Here's the drawing with two shaded views (mm, measured from the low corner). I have some questions. Coordinates: 2 decimals unless noted, no trailing zeros. Loops run counter-clockwise (first coordinate to the right, second up) from the corner with the lowest first, then second, coordinate; pieces in that order, holes last. Notation, with made-up numbers: M 70.25,7.25 L 80.25,7.25 A13 ccw 80.25,21.25 Z; hole C 38,5 d4. An arc over 180 degrees is marked long. Return JSON: item names as keys, results as strings. Group by question number.
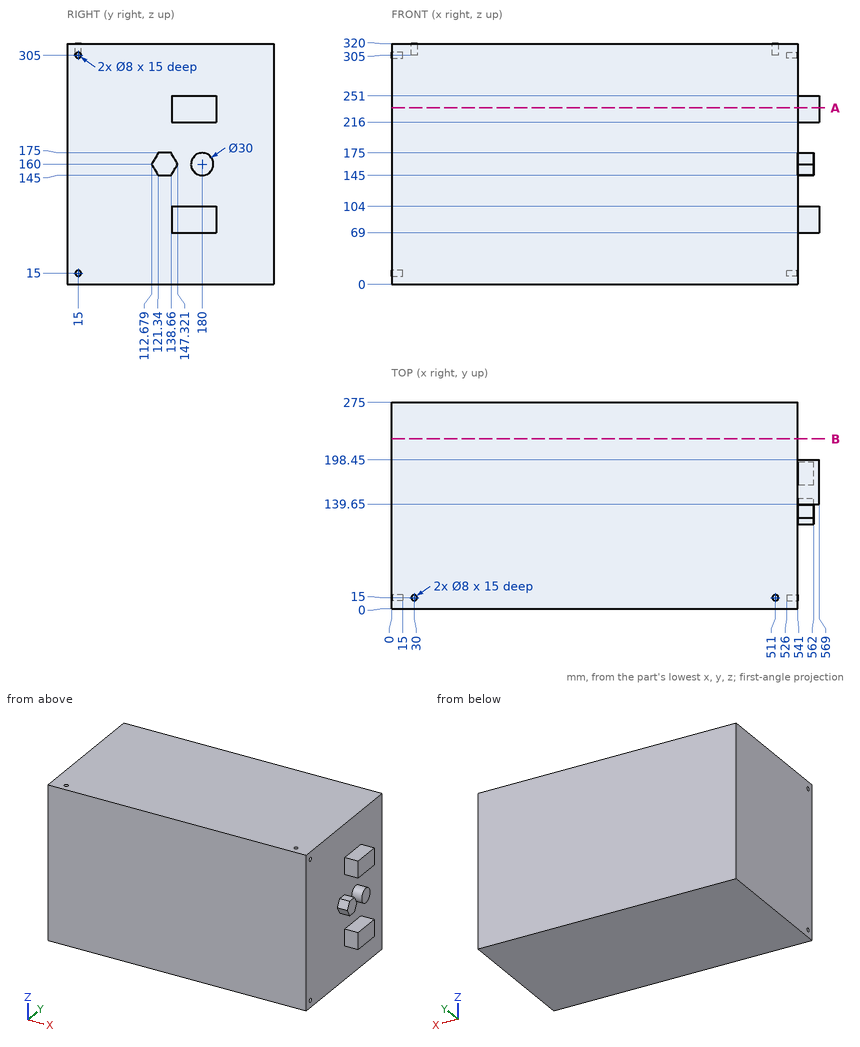
1) For pin 1 (8.5 mm diameter, centred on x = 551, z = 239.5, fed in from +Y); pin 2 (6 mm diameter, centred on x = 210.5, y = 198.5, fed in from -Z); pin 3 (7 mm diameter, centred on y = 15, z = 305, fed in from +X); pin 4 (10 mm diameter, centred on y = 240.5, z = 159.5, fed in from +X), each with a flat end and sliding along its axis, tell me the tip position at first contact or that it passes through.
2) Suppose I cut it at B-B, the plane y = 226.5. List the corners of the cut face in (x, z) for me.
3) If I drill on line 1 (Y direction, x = 6, z = 305); line 2 (X direction, y = 163, z = 214), over which ranges is the centre line in solid material (lowest first)? Write a range as from..to.
4) Suppose I cut it at A-A, the plane z = 235. List the corners of the cut face in (x, y) for me.
Returned:
{
 "1": {"pin 1": "stops at y = 198.45", "pin 2": "stops at z = 0", "pin 3": "stops at x = 526", "pin 4": "stops at x = 541"},
 "2": {"outline": "M 0,0 L 541,0 L 541,320 L 0,320 Z"},
 "3": {"line 1": "y = 0..11, 19..275", "line 2": "x = 0..541"},
 "4": {"outline": "M 0,0 L 541,0 L 541,139.65 L 569,139.65 L 569,198.45 L 541,198.45 L 541,275 L 0,275 Z"}
}
